from build123d import *

# Parameters (mm, degrees)
F1_DEPTH = 12.7
F2_DEPTH = 95.25


# Not quite as in the source:
# - a feature names something its author has since deleted; it is built from what else it names


with BuildPart() as f1:
    # F0 (on Front) → F1 (new body)
    with BuildSketch(Plane.XZ):
        Polygon((-4.278267482, -28.4575006988), (-22.6091385288, 3.2924993012), (-59.2708806223, 3.2924993012), (-77.6017516691, -28.4575006988), (-59.2708806223, -60.2075006988), (-22.6091385288, -60.2075006988), align=None)
        Polygon((-57.4377935176, -57.0325006988), (-73.9355774597, -28.4575006988), (-57.4377935176, 0.1174993012), (-24.4422256334, 0.1174993012), (-7.9444416913, -28.4575006988), (-24.4422256334, -57.0325006988), align=None, mode=Mode.SUBTRACT)
        Polygon((-22.6091385288, 3.2924993012), (-4.278267482, 35.0424993012), (-22.6091385288, 66.7924993012), (-27.4963065598, 66.7924993012), (-59.2708806223, 66.7924993012), (-77.6017516691, 35.0424993012), (-59.2708806223, 3.2924993012), align=None)
        Polygon((-57.4377935176, 6.4674993012), (-73.9355774597, 35.0424993012), (-57.4377935176, 63.6174993012), (-24.4422256334, 63.6174993012), (-7.9444416913, 35.0424993012), (-24.4422256334, 6.4674993012), align=None, mode=Mode.SUBTRACT)
        Polygon((-22.6091385288, 66.7924993012), (-4.278267482, 35.0424993012), (27.4963065701, 35.0424993012), (32.3834746115, 35.0424993012), (50.7143456583, 66.7924993012), (32.3834746115, 98.5424993012), (-4.278267482, 98.5424993012), align=None)
        Polygon((-2.4451803773, 38.2174993012), (-18.9429643194, 66.7924993012), (-2.4451803773, 95.3674993012), (30.5503875069, 95.3674993012), (47.048171449, 66.7924993012), (30.5503875069, 38.2174993012), align=None, mode=Mode.SUBTRACT)
        Polygon((-2.4451803773, 95.3674993012), (-18.9429643194, 66.7924993012), (-2.4451803773, 38.2174993012), (30.5503875069, 38.2174993012), (47.048171449, 66.7924993012), (30.5503875069, 95.3674993012), align=None)
        Polygon((-57.4377935176, 0.1174993012), (-73.9355774597, -28.4575006988), (-57.4377935176, -57.0325006988), (-24.4422256334, -57.0325006988), (-7.9444416913, -28.4575006988), (-24.4422256334, 0.1174993012), align=None)
        Polygon((-57.4377935176, 63.6174993012), (-73.9355774597, 35.0424993012), (-57.4377935176, 6.4674993012), (-24.4422256334, 6.4674993012), (-7.9444416913, 35.0424993012), (-24.4422256334, 63.6174993012), align=None)
    extrude(amount=F1_DEPTH)

    # F0 (on Front) → F2 (join)
    with BuildSketch(Plane.XZ):
        Polygon((-22.6091385288, 3.2924993012), (-4.278267482, 35.0424993012), (-22.6091385288, 66.7924993012), (-27.4963065598, 66.7924993012), (-59.2708806223, 66.7924993012), (-77.6017516691, 35.0424993012), (-59.2708806223, 3.2924993012), align=None)
        Polygon((-57.4377935176, 6.4674993012), (-73.9355774597, 35.0424993012), (-57.4377935176, 63.6174993012), (-24.4422256334, 63.6174993012), (-7.9444416913, 35.0424993012), (-24.4422256334, 6.4674993012), align=None, mode=Mode.SUBTRACT)
        Polygon((-22.6091385288, 66.7924993012), (-4.278267482, 35.0424993012), (27.4963065701, 35.0424993012), (32.3834746115, 35.0424993012), (50.7143456583, 66.7924993012), (32.3834746115, 98.5424993012), (-4.278267482, 98.5424993012), align=None)
        Polygon((-2.4451803773, 38.2174993012), (-18.9429643194, 66.7924993012), (-2.4451803773, 95.3674993012), (30.5503875069, 95.3674993012), (47.048171449, 66.7924993012), (30.5503875069, 38.2174993012), align=None, mode=Mode.SUBTRACT)
        Polygon((-4.278267482, -28.4575006988), (-22.6091385288, 3.2924993012), (-59.2708806223, 3.2924993012), (-77.6017516691, -28.4575006988), (-59.2708806223, -60.2075006988), (-22.6091385288, -60.2075006988), align=None)
        Polygon((-57.4377935176, -57.0325006988), (-73.9355774597, -28.4575006988), (-57.4377935176, 0.1174993012), (-24.4422256334, 0.1174993012), (-7.9444416913, -28.4575006988), (-24.4422256334, -57.0325006988), align=None, mode=Mode.SUBTRACT)
        Polygon((27.4963065701, 35.0424993012), (-4.278267482, 35.0424993012), (-22.6091385288, 3.2924993012), (-4.278267482, -28.4575006988), (-22.6091385288, -60.2075006988), (-59.2708806223, -60.2075006988), (-57.4378374826, -63.3825006988), (-20.7760404334, -63.3825006988), (-0.612082282, -28.4575006988), (-18.9429533288, 3.2924993012), (-2.4451693867, 31.8674993012), (30.5503875069, 31.8674993012), (32.3834746115, 35.0424993012), align=None)
        Polygon((-27.4963065598, 66.7924993012), (-22.6091385288, 66.7924993012), (-4.278267482, 98.5424993012), (-7.9444416913, 98.5424993012), (-24.4422256334, 69.9674993012), (-57.4377935176, 69.9674993012), (-59.2708806223, 66.7924993012), align=None)
    extrude(amount=F2_DEPTH)


solid = f1.part
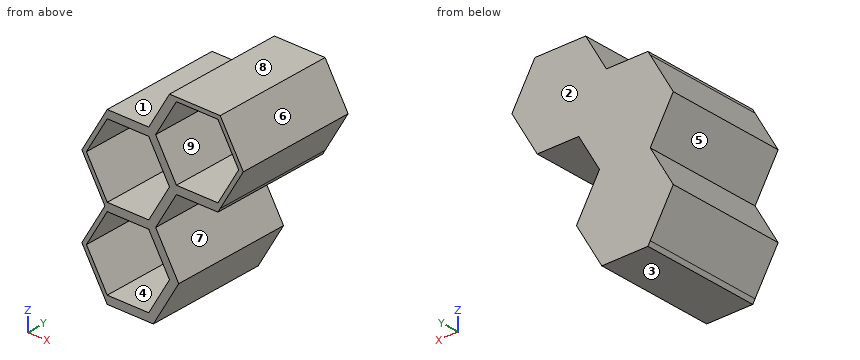
Source: CAD feature listing. Evaluate the final solid. Frame: model axes, mm. Face numbers are marked on the shaded views. A direction names the side the tool comes from. Give positions to 0.01 mm unless a question says otherwise; leave off trailing zeros. Write each loop counter-clockwise with the first axis right and the second up, starting at its lowest first coordinate (ties: lowest second). Pieces come first, ordered by that corner, then holes. Notation, with made-up numbers: M 84,-19 L 95,-19 A25 cw 95,18 Z; hole C 66.25,-30 d8. An arc over 180 degrees is marked long. Return JSON: item names as keys, results as strings. Group by question number.
1) Set-up query: the marked faces 5, 6, 7, 8 and 9. Return all of +Z, -Z, +X, -X, +Y, -Y with unobstructed straight access to the full face (end or side cutting, diameter ignored); none if empty.
2) Cut plane D-D, the plane x = -65. Output: boundary loops of the cut face in (y, z).
3) Cut plane C-C, the plane z = 24.5. Output: boundary loops of the cut face in (x, y), then the cut area to 3 significant figures.
4) First-contact query: pin 1 Ø3 at (x, z) = (-15.5, 38) entering from -Y; pin 2 Ø10 at (y, z) = (-32.5, 65.5) entering from -X; pin 3 Ø12 at (x, z) = (22.5, 44) entering from +Y; pin 4 Ø10 at (x, y) = (-40, -64.5) entering from +Z. Flat tips, straight axial feed; report the tip coordinate or a pass-through.
5) Draft query along Z for the marked faces 1, 2, 3 and 4. Return one class per face: released by +Z, released by -Z, zero draft, split by the parting line, or undercut.
6) Ray query, L1, parallel to Z at x = -29.5, y = -30; L2, parallel to X at y = -80, z = 49.5; L3, parallel to Z at x = -61.5, y = -62. Return the intervals inside material, ascending.
7) Cut plane A-A, the plane x = -51. Output: boundary loops of the cut face in (y, z).
8) Cut plane B-B, the plane y = -8. Output: boundary loops of the cut face in (x, z), then the cut area to 3 significant figures.
Data:
{
 "1": {"face 5": "-X, +Y, -Y", "face 6": "+Z, +X, +Y, -Y", "face 7": "+X, +Y, -Y", "face 8": "+Z, +X, -X, +Y, -Y", "face 9": "-Y"},
 "2": {"outline": "M -95.25,-50.28 L 0,-50.28 L 0,-6.63 L -95.25,-6.63 L -95.25,-12.98 L -12.7,-12.98 L -12.7,-43.93 L -95.25,-43.93 Z; M -95.25,13.22 L 0,13.22 L 0,56.87 L -95.25,56.87 L -95.25,50.52 L -12.7,50.52 L -12.7,19.57 L -95.25,19.57 Z"},
 "3": {"outline": "M -71.52,-95.25 L -67.85,-95.25 L -67.85,-12.7 L -14.03,-12.7 L -14.03,-95.25 L -6.7,-95.25 L -6.7,0 L -71.52,0 Z", "area": "1,730 mm²"},
 "4": {"pin 1": "stops at y = -12.7", "pin 2": "stops at x = -62.9", "pin 3": "stops at y = 0", "pin 4": "stops at z = 69.97"},
 "5": {"face 1": "released by +Z", "face 2": "zero draft", "face 3": "released by -Z", "face 4": "undercut"},
 "6": {"L1": "z = -63.38 to -57.03, 0.12 to 6.47, 63.62 to 69.97", "L2": "x = -69.25 to -65.59, -16.29 to -8.96, 37.06 to 40.73", "L3": "z = -56.35 to -50, -6.92 to -0.57, 7.15 to 13.5, 56.58 to 62.93"},
 "7": {"outline": "M -95.25,-63.38 L 0,-63.38 L 0,69.97 L -95.25,69.97 L -95.25,63.62 L -12.7,63.62 L -12.7,6.47 L -95.25,6.47 L -95.25,0.12 L -12.7,0.12 L -12.7,-57.03 L -95.25,-57.03 Z"},
 "8": {"outline": "M -77.6,-28.46 L -59.27,-60.21 L -57.44,-63.38 L -20.78,-63.38 L -0.61,-28.46 L -18.94,3.29 L -2.45,31.87 L 30.55,31.87 L 50.71,66.79 L 32.38,98.54 L -7.94,98.54 L -24.44,69.97 L -57.44,69.97 L -77.6,35.04 L -59.27,3.29 Z", "area": "11,300 mm²"}
}
